```python
from build123d import *

# Parameters (mm, degrees)
SKETCH_2_R            = 11
EXTRUDE_1_DEPTH       = 2
SKETCH_7_R            = 5
EXTRUDE_2_DEPTH       = 10
CUT_EXTRUDE_3_REACH   = 21.647
SKETCH_8_R            = 2
HOLE_WIZARD_M31_D     = 3.15
HOLE_WIZARD_M31_DEPTH = 8
HOLE_WIZARD_M31_TIP   = 0.946355475
SKETCH_12_R           = 1.5
CUT_EXTRUDE_4_DEPTH   = 10


with BuildPart() as part:
    # Эскиз2 → Бобышка-Вытянуть1 (new body)
    with BuildSketch(Plane(origin=(0, 0, 0), x_dir=(1, 0, 0), z_dir=(0, 1, 0))):
        with Locations(Location((0, 0, 0), (0, 0, 270))):
            Circle(SKETCH_2_R)
    extrude(amount=EXTRUDE_1_DEPTH)

    # Эскиз7 → Бобышка-Вытянуть2 (add)
    with BuildSketch(Plane(origin=(0, 2, 0), x_dir=(1, 0, 0), z_dir=(0, 1, 0))):
        with Locations(Location((0, 0, 0), (0, 0, 270))):
            Circle(SKETCH_7_R)
    extrude(amount=EXTRUDE_2_DEPTH)

    # Эскиз8 → Вырез-Вытянуть3 (cut, up to next)
    with BuildSketch(Plane(origin=(0, 12, 0), x_dir=(1, 0, 0), z_dir=(0, 1, 0)), mode=Mode.PRIVATE) as cut_extrude_3_sk1:
        with Locations(Location((0, 0, 0), (0, 0, 270))):
            Circle(SKETCH_8_R)
    cut_extrude_3_tool1 = extrude(cut_extrude_3_sk1.sketch, amount=-CUT_EXTRUDE_3_REACH, mode=Mode.PRIVATE) & part.part
    add(cut_extrude_3_tool1.solids().sort_by_distance((0, 12, 0))[0], mode=Mode.SUBTRACT)

    # Сверло под метчик  спиральное M31
    with Locations(Plane(origin=(0, 2, 0), x_dir=(1, 0, 0), z_dir=(0, 1, 0))):
        with Locations((0, -8), (-8, 0), (0, 8.225054206), (8, 0)):
            Hole(HOLE_WIZARD_M31_D / 2, depth=HOLE_WIZARD_M31_DEPTH)
            with Locations((0, 0, -(HOLE_WIZARD_M31_DEPTH + HOLE_WIZARD_M31_TIP / 2))):  # 118° drill point
                Cone(0, HOLE_WIZARD_M31_D / 2, HOLE_WIZARD_M31_TIP, mode=Mode.SUBTRACT)

    # Эскиз12 → Вырез-Вытянуть4 (cut)
    with BuildSketch(Plane.XY):
        with Locations((0, 7)):
            Circle(SKETCH_12_R)
    extrude(amount=-CUT_EXTRUDE_4_DEPTH, mode=Mode.SUBTRACT)


solid = part.part
```
Geometry: final body of the model. Coordinates: model frame, mm. A direction names the side the tool comes from. Round coordinates to 2 decimals unless told otherwise and drop trailing zeros. Write each loop counter-clockwise with the first axis right and the second up, starting at its lowest first coordinate (ties: lowest second). Pieces come first, ordered by that corner, then holes. Notation, with made-up numbers: M 48.5,-28.5 L 89.5,-28.5 A28 cw 89.5,-9.5 Z; hole C -28.5,-31 d10. An arc over 180 degrees is marked long. Answer in a Markdown table with one row per item. Add a question column.
(1) Contact query for flat-ended pins moving along their axis: pin 1 (1.9 mm diameter, centred on x = -8, z = 0, fed in from -Y); pin 2 (3 mm diameter, centred on x = -6, z = 8, fed in from +Y); pin 3 (2.5 mm diameter, centred on x = 0, y = 7, fed in from -Z); pin 4 (1 mm diameter, centred on y = 8.5, z = -3.5, fed in from -X). Output: stop coordinate, or through.
(2) Cut plane B-B, the plane z = 0. Return the cut outline in (x, y) (3 decimals), then the cut area to 3 significant figures.
(3) Ray query, L1, parallel to Z at x = 1.5, y = 10.25; L2, parallel to Z at x = 1.75, y = 10; L3, parallel to Y at x = 6.25, z = 5.25. Return the intervals inside material, ascending.
(4) Draft query along X for faces 1 (the face through (9.573, 0.986, -0.069)), 2 (the face through (1.5, 6.93, 4.77)), 3 (the face through (-5, 2, 2)), 4 (the face through (-0.766, 6.084, 1.847)). Return one class per face: pulls with the +X half, pulls with the -X half, needs draft (parallel to the pull), parting line crosses it, or undercut.
(5) Cut plane C-C, the plane x = -8. Return the cut outline in (y, z) (3 decimals), then the cut area to 3 significant figures.
(6) Reachability of faces 5 (the face through (-6.427, 0.986, -0.069)), 6 (the face through (1.43, 7.45, -3.14)) from +Z, -Z, +X, -X, +Y, -Y: full face, straight path, thin tool, end or side. Return the list, or none.
(7) Cut plane A-A, the plane x = 0. Return the cut outline in (y, z) (3 decimals), then the cut area to 3 significant figures.
(8) Cut plane D-D, the plane z = -4. Return the cut outline in (x, y).
Established:
| question | item | result |
|---|---|---|
| 1 | pin 1 | through |
| 1 | pin 2 | y = 2 |
| 1 | pin 3 | z = 1.56 |
| 1 | pin 4 | x = -4 |
| 2 | outline | M -11,0 L -9.575,0 L -9.575,2 L -11,2 Z; M -6.425,0 L -2,0 L -2,12 L -5,12 L -5,2 L -6.425,2 Z; M 2,0 L 6.425,0 L 6.425,2 L 5,2 L 5,12 L 2,12 Z; M 9.575,0 L 11,0 L 11,2 L 9.575,2 Z |
| 2 | area | 83.4 mm² |
| 3 | L1 | -4.77 to -1.32, 1.32 to 4.77 |
| 3 | L2 | -4.68 to -0.97, 0.97 to 4.68 |
| 3 | L3 | 0 to 2 |
| 4 | face 1 | undercut |
| 4 | face 2 | parting line crosses it |
| 4 | face 3 | needs draft |
| 4 | face 4 | undercut |
| 5 | outline | M 0,-7.55 L 2,-7.55 L 2,-1.575 L 0,-1.575 Z; M 0,1.575 L 2,1.575 L 2,7.55 L 0,7.55 Z |
| 5 | area | 23.9 mm² |
| 6 | face 5 | +Y, -Y |
| 6 | face 6 | -Z |
| 7 | outline | M 0,-11 L 2,-11 L 2,-9.8 L 0,-9.8 Z; M 0,-6.65 L 2,-6.65 L 2,-5 L 5.5,-5 L 5.5,-2 L 0,-2 Z; M 0,2 L 12,2 L 12,5 L 2,5 L 2,6.425 L 0,6.425 Z; M 0,9.575 L 2,9.575 L 2,11 L 0,11 Z; M 8.5,-5 L 12,-5 L 12,-2 L 8.5,-2 Z |
| 7 | area | 74.4 mm² |
| 8 | outline | M -10.25,0 L 10.25,0 L 10.25,2 L 3,2 L 3,12 L -3,12 L -3,2 L -10.25,2 Z; hole C 0,7 d3 |
